Read the model definition and answer for the solid it produces. Units are mm, in the model's axes. Coordinates: 2 decimals unless noted, no trailing zeros. Write each loop counter-clockwise with the first axis right and the second up, starting at its lowest first coordinate (ties: lowest second). Pieces come first, ordered by that corner, then holes. Notation, with made-up numbers: (73.25, 87.25) - (127.25, 87.25) arc R26 ccw to (127.25, 106.25) - close; hole circle Ø11 at (-31.75, 10). An arc over 180 degrees is marked (long way). Use a Markdown table: item, result.
from build123d import *

# Parameters (mm, degrees)
SKETCH1_W           = 229
SKETCH1_H           = 149.5
BOSS_EXTRUDE1_DEPTH = 3.2
SKETCH2_W           = 229
SKETCH2_H           = 22
BOSS_EXTRUDE2_DEPTH = 5
SKETCH3_W           = 26.5
SKETCH3_H           = 8.8
SKETCH3_W_2         = 11
SKETCH3_H_2         = 114.3
BOSS_EXTRUDE3_DEPTH = 3
SKETCH4_R           = 2
BOSS_EXTRUDE4_DEPTH = 10


with BuildPart() as part:
    # Sketch1 → Boss-Extrude1 (new body)
    with BuildSketch(Plane(origin=(0, 0, 0), x_dir=(1, 0, 0), z_dir=(0, 1, 0))):
        Rectangle(SKETCH1_W, SKETCH1_H)
    extrude(amount=BOSS_EXTRUDE1_DEPTH)

    # Sketch2 → Boss-Extrude2 (add)
    with BuildSketch(Plane(origin=(0, 3.2, 0), x_dir=(1, 0, 0), z_dir=(0, 1, 0))):
        with Locations((0, -63.75)):
            Rectangle(SKETCH2_W, SKETCH2_H)
    extrude(amount=-BOSS_EXTRUDE2_DEPTH)

    # Sketch3 → Boss-Extrude3 (add)
    with BuildSketch(Plane.XZ.offset(1.8)):
        Polygon((-41, 52.75), (-67.5, 52.75), (-67.5, 39.55), (-59.75, 39.55), (-48.75, 39.55), (-41, 39.55), align=None)
        with Locations((-54.25, 57.15)):
            Rectangle(SKETCH3_W, SKETCH3_H)
        with Locations((-54.25, -17.6)):
            Rectangle(SKETCH3_W_2, SKETCH3_H_2)
    extrude(amount=BOSS_EXTRUDE3_DEPTH)

    # Sketch4 → Boss-Extrude4 (add)
    with BuildSketch(Plane(origin=(0, 0, -74.75), x_dir=(-1, 0, 0), z_dir=(0, 0, -1))):
        with Locations(Location((54.25, -3.3, 0), (0, 0, 131.409622109))):
            Circle(SKETCH4_R)
    extrude(amount=BOSS_EXTRUDE4_DEPTH)


solid = part.part
(1) A cutting plane is placed at B-B, the plane y = -3.3. Write down the section's boundary in (x, z), and give its area (3 significant figures).
Report:
| item | result |
|---|---|
| outline | (-67.5, 39.55) - (-59.75, 39.55) - (-59.75, -74.75) - (-56.25, -74.75) - (-56.25, -84.75) - (-52.25, -84.75) - (-52.25, -74.75) - (-48.75, -74.75) - (-48.75, 39.55) - (-41, 39.55) - (-41, 61.55) - (-67.5, 61.55) - close |
| area | 1,880 mm² |
(2) A cutting plane is placed at A-A, the plane z = -56. Write down the section's boundary in (x, y).
Report:
| item | result |
|---|---|
| outline | (-114.5, 0) - (114.5, 0) - (114.5, 3.2) - (-114.5, 3.2) - close; (-59.75, -4.8) - (-48.75, -4.8) - (-48.75, -1.8) - (-59.75, -1.8) - close |
(3) A cutting plane is placed at D-D, the plane x = 25.5. Write down the section's boundary in (y, z).
Report:
| item | result |
|---|---|
| outline | (-1.8, 52.75) - (0, 52.75) - (0, -74.75) - (3.2, -74.75) - (3.2, 74.75) - (-1.8, 74.75) - close |
(4) Straight lines are drawn through the part: L1, parallel to Z at x = 90.5, y = -1.5; L2, parallel to Y at x = -84, z = 48; L3, parallel to Z at x = 92, y = 2.5. For each, find the intervals that lie inside material, in ascending order.
Report:
| item | result |
|---|---|
| L1 | z = 52.75 to 74.75 |
| L2 | y = 0 to 3.2 |
| L3 | z = -74.75 to 74.75 |
(5) The mould has two halves that part along Y. Classify faces 1 (the flat face through (-2, 1, 74.75)), 2 (the flat face through (-54, -4.8, 9)), 3 (the flat face through (-2, 3.2, -1)), 4 (the flat face through (-54, -1.8, 4)): pulls with the +Y half, pulls with the -Y half, needs draft (parallel to the pull), parting line crosses it, or undercut.
Report:
| item | result |
|---|---|
| face 1 | needs draft |
| face 2 | pulls with the -Y half |
| face 3 | pulls with the +Y half |
| face 4 | undercut |
(6) A cutting plane is placed at C-C, the plane x = -64.5. Write down the section's boundary in (y, z), and give its area (3 significant figures).
Report:
| item | result |
|---|---|
| outline | (-4.8, 39.55) - (-1.8, 39.55) - (-1.8, 52.75) - (0, 52.75) - (0, -74.75) - (3.2, -74.75) - (3.2, 74.75) - (-1.8, 74.75) - (-1.8, 61.55) - (-4.8, 61.55) - close |
| area | 584 mm² |
(7) Each of these flat-tipped pins is pushed along its axis until it touches: P1, Ø0.9, axis at y = -3, z = 54.5, coming from the +X side; P2, Ø1, axis at x = 43, y = 1, coming from the -Z side; P3, Ø0.9, axis at y = -3.5, z = -1, coming from the +X side; P4, Ø1.5, axis at x = -52, y = -3, coming from the -Z side. Where does it stop, or does it pass through?
Report:
| item | result |
|---|---|
| P1 | stops at x = -41 |
| P2 | stops at z = -74.75 |
| P3 | stops at x = -48.75 |
| P4 | stops at z = -84.75 |
